Autodesk Inventor part; units mm, degrees
ref_plane "COMBINATION_MODULE_XY" through (0, 0, 0) normal (1, 0, 0) x (0, 0, -1)
ref_plane "COMBINATION_MODULE_YZ" through (0, 0, 0) normal (0, 0, -1) x (0, 1, 0)
ref_plane "COMBINATION_MODULE_ZX" through (0, 0, 0) normal (0, 1, 0) x (1, 0, 0)
sketch "Sketch_1" plane through (0, 0, 0) normal (0, 0, 1) x (1, 0, 0)
  line L0 (74, 0) -> (0, 0)
  line L1 (0, 0) -> (0, 4.5)
  line L2 (0, 4.5) -> (0.5, 5)
  line L3 (0.5, 5) -> (73.5, 5)
  line L4 (73.5, 5) -> (74, 4.5)
  line L5 (74, 4.5) -> (74, 0)
  line L6 (74, 0) -> (0, 0)
revolve "Revolution1" add sketch "Sketch_1" angle 360 about axis through (74, 0, 0) along (1, 0, 0)
sketch "_____10" plane through (0, 0, 5) normal (0, 0, 1) x (1, 0, 0)
  arc A0 (33, 1.5) -> (33, -1.5) centre (33, 0) ccw
  line L0 (33, -1.5) -> (41, -1.5)
  arc A1 (41, -1.5) -> (41, 1.5) centre (41, 0) ccw
  line L1 (41, 1.5) -> (33, 1.5)
extrude "Extrusion1" cut sketch "_____10" against normal blind 1.8
sketch "_____5" plane through (3, 0, 0) normal (1, 0, 0) x (0, 0, -1)
  circle A0 centre (0, 0) radius 10
  circle A1 centre (0, 0) radius 4.8
extrude "Extrusion2" cut sketch "_____5" against normal blind 1.15
sketch "_____6" plane through (71, 0, 0) normal (1, 0, 0) x (0, 0, -1)
  circle A0 centre (0, 0) radius 10
  circle A1 centre (0, 0) radius 4.8
extrude "Extrusion3" cut sketch "_____6" along normal blind 1.15
ref_plane "COMBINATION_MODULE_XY" through (0, 0, 0) normal (1, 0, 0) x (0, 0, -1)
ref_plane "COMBINATION_MODULE_YZ" through (0, 0, 0) normal (0, 0, -1) x (0, 1, 0)
ref_plane "COMBINATION_MODULE_ZX" through (0, 0, 0) normal (0, 1, 0) x (1, 0, 0)
ref_plane "to_ring_b_XY" through (2.425, 0, 0) normal (1, 0, 0) x (0, 0, -1)
ref_plane "to_ring_b_YZ" through (2.425, 0, 0) normal (0, 0, -1) x (0, 1, 0)
ref_plane "to_ring_b_ZX" through (2.425, 0, 0) normal (0, 1, 0) x (1, 0, 0)
ref_plane "to_ring_s_XY" through (71.575, 0, 0) normal (1, 0, 0) x (0, 0, -1)
ref_plane "to_ring_s_YZ" through (71.575, 0, 0) normal (0, 0, -1) x (0, 1, 0)
ref_plane "to_ring_s_ZX" through (71.575, 0, 0) normal (0, 1, 0) x (1, 0, 0)
properties part number "NSFMRRA10-74-B3-S3-KC31.5-A11(000_000)_s"
Check sheet for the modelled part. Datum: model origin and axes. Units: mm. A direction names the side the tool comes from. Give positions to 0.01 mm unless a question says otherwise; leave off trailing zeros. Loops run counter-clockwise (first coordinate to the right, second up) from the corner with the lowest first, then second, coordinate; pieces in that order, holes last. Notation, with made-up numbers: M -35,71.25 L -22,71.25 A7 cw -22,77.25 Z; hole C -7.75,64.5 d9. An arc over 180 degrees is marked long. Return JSON: item names as keys, results as strings. Group by question number.
1. Go/stop test with flat-tipped pins: pin 1 (2.5 mm diameter, centred on x = 39.5, y = -0.5, fed in from +Z); pin 2 (1 mm diameter, centred on x = 28, y = -3, fed in from +Z); pin 3 (0.5 mm diameter, centred on x = 38.5, z = 4, fed in from -Y). Record where each tip stops, or that it passes through.
2. Thickness scan on L1, parallel to Z at x = 56.5, y = -0.25; L2, parallel to Z at x = 47.5, y = -0.75; L3, parallel to Y at x = 16.5, z = 2.25. Record the ranges inside material, lowest first.
3. Tool access check on faces 1 (the flat face through (37, 0, 3.2)), 2 (the cylindrical face through (2.43, 4.05, -2.58)), 3 (the cylindrical face through (1.18, -1.08, -4.88)). Record the directions out of +Z, -Z, +X, -X, +Y, -Y that give a thin tool (end or side, any length) a straight path to the whole face; none if there is none.
4. Cross-section at A-A on y = 0. Record the boundary of the cut face in (x, z), plus the area to 3 significant figures.
5. Mould release check, pull along Y, two halves, no side actions. Record for faces 4 (the flat face through (37, 1.5, 4)), 5 (the cylindrical face through (71.57, -4.05, -2.58)), 6 (the flat face through (0, 0, 0)), 7 (the cylindrical face through (31.5, 0, 4.1)): released by +Y, released by -Y, zero draft, split by the parting line, or undercut.
6. Cross-section at B-B on x = 61. Record the boundary of the cut face in (y, z).
Return value:
{
 "1": {"pin 1": "z = 4.77", "pin 2": "z = 4.33", "pin 3": "y = -3.31"},
 "2": {"L1": "-4.99 to 4.99", "L2": "-4.94 to 4.94", "L3": "-4.47 to 4.47"},
 "3": {"face 1": "+Z", "face 2": "none", "face 3": "+X, -X"},
 "4": {"outline": "M 0,-4.5 L 0.5,-5 L 1.85,-5 L 1.85,-4.8 L 3,-4.8 L 3,-5 L 71,-5 L 71,-4.8 L 72.15,-4.8 L 72.15,-5 L 73.5,-5 L 74,-4.5 L 74,4.5 L 73.5,5 L 72.15,5 L 72.15,4.8 L 71,4.8 L 71,5 L 42.5,5 L 42.5,3.2 L 31.5,3.2 L 31.5,5 L 3,5 L 3,4.8 L 1.85,4.8 L 1.85,5 L 0.5,5 L 0,4.5 Z", "area": "719 mm^2"},
 "5": {"face 4": "undercut", "face 5": "split by the parting line", "face 6": "zero draft", "face 7": "undercut"},
 "6": {"outline": "C 0,0 d10"}
}
